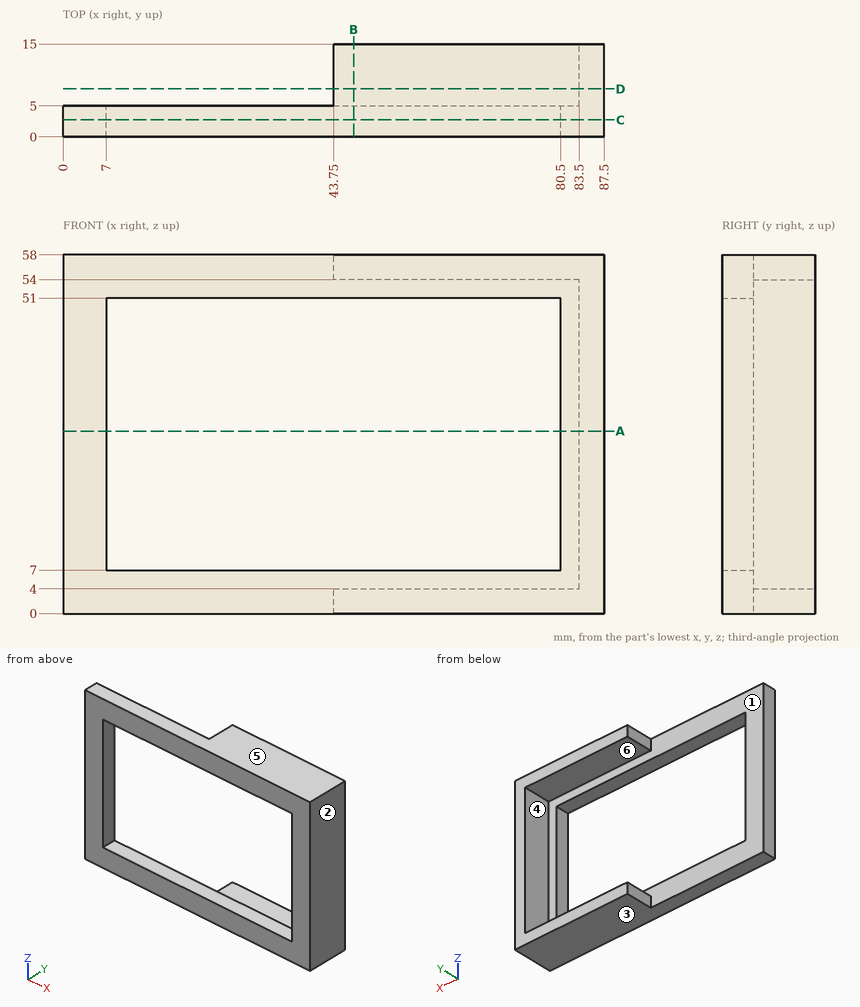
Verification items for this drawing (mm, ordinates from the low corner). A direction names the side the tool comes from. Round coordinates to 2 decimals unless told otherwise and drop trailing zeros. Write each loop counter-clockwise with the first axis right and the second up, starting at its lowest first coordinate (ties: lowest second). Pieces come first, ordered by that corner, then holes. Notation, with made-up numbers: (40, 30.5) - (44, 30.5) arc R17 ccw to (44, 35.5) - close; hole circle Ø7 at (64.25, 45). An arc over 180 degrees is marked (long way). One line per item, written item: value.
1. Cross-section at A-A on z = 29.5. Record the boundary of the cut face in (x, y).
The answers:
outline: (0, 0) - (7, 0) - (7, 5) - (0, 5) - close; (80.5, 0) - (87.5, 0) - (87.5, 15) - (83.5, 15) - (83.5, 5) - (80.5, 5) - close
2. Cross-section at B-B on x = 47. Record the boundary of the cut face in (y, z).
The answers:
outline: (0, 0) - (15, 0) - (15, 4) - (5, 4) - (5, 7) - (0, 7) - close; (0, 51) - (5, 51) - (5, 54) - (15, 54) - (15, 58) - (0, 58) - close
3. Mould release check, pull along Z, two halves, no side actions. Record for the marked faces 1, 2, 3 and 4: released by +Z, released by -Z, zero draft, split by the parting line, or undercut.
The answers:
face 1: undercut
face 2: zero draft
face 3: released by -Z
face 4: undercut
4. Cross-section at C-C on y = 2.75. Record the boundary of the cut face in (x, z).
The answers:
outline: (0, 0) - (87.5, 0) - (87.5, 58) - (0, 58) - close; hole (7, 7) - (80.5, 7) - (80.5, 51) - (7, 51) - close
5. Scan lines: L1, parallel to Z at x = 31.5, y = 2.75; L2, parallel to X at y = 2.75, z = 46.5; L3, parallel to Z at x = 57, y = 14.25. Record each from-to range of solid material in increasing order.
The answers:
L1: z = 0 to 7, 51 to 58
L2: x = 0 to 7, 80.5 to 87.5
L3: z = 0 to 4, 54 to 58
6. Set-up check for the marked faces 5 and 6: record each of +Z, -Z, +X, -X, +Y, -Y from which the full face is reachable in a straight line by a thin tool's end or side.
The answers:
face 5: +Z, +X, -X, +Y, -Y
face 6: -X, +Y
7. Cross-section at D-D on y = 7.75. Record the boundary of the cut face in (x, z).
The answers:
outline: (43.75, 0) - (87.5, 0) - (87.5, 58) - (43.75, 58) - (43.75, 54) - (83.5, 54) - (83.5, 4) - (43.75, 4) - close
8. Depth check by flat-ended pin: pin 1 Ø8 at (x, y) = (71.5, 5) entering from -Z; pin 2 Ø3 at (y, z) = (8.5, 55) entering from -X; pin 3 Ø5 at (y, z) = (9.5, 20.5) entering from -X. Enter the tip coordinate at first touch or a pass-through.
The answers:
pin 1: stops at z = 0
pin 2: stops at x = 43.75
pin 3: stops at x = 83.5
